For this review, use the dimensioned drawing (mm, ordinates from the lowest corner) and the shaded views. Give positions to 0.01 mm unless a question says otherwise; leave off trailing zeros. Order: outer loops, then holes, each group sorted by start corner. A loop starts at its lowest first (then second) coordinate and runs counter-clockwise, first axis right, second up.
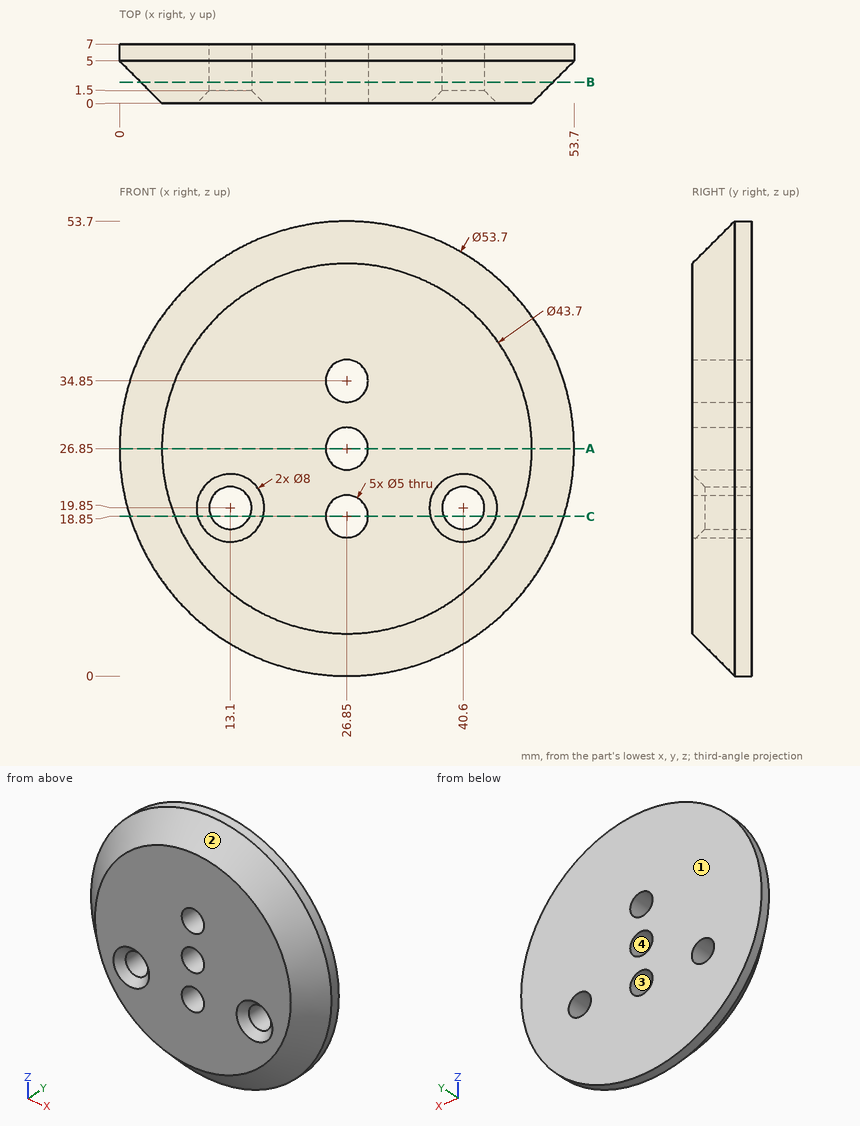
1. Take a section at A-A (z = 26.85). State the section outline as (x, y) points, then the cut area to 3 significant figures.
Recorded:
outline: (0, 5) - (5, 0) - (24.35, 0) - (24.35, 7) - (0, 7) - close; (29.35, 0) - (48.7, 0) - (53.7, 5) - (53.7, 7) - (29.35, 7) - close
area: 316 mm2
2. For pin 1 (3 mm diameter, centred on x = 26.85, z = 34.85, fed in from +Y), flat-tipped, find the tip position at first contact; note if it passes through.
Recorded:
pin 1: passes through
3. Take a section at B-B (y = 2.5). State the section outline as (x, z) points, then the cut area to 3 significant figures.
Recorded:
outline: circle Ø48.7 at (26.85, 26.85); hole circle Ø5 at (13.1, 19.85); hole circle Ø5 at (26.85, 18.85); hole circle Ø5 at (26.85, 26.85); hole circle Ø5 at (26.85, 34.85); hole circle Ø5 at (40.6, 19.85)
area: 1,760 mm2
4. For line 1 along Z through (x, y) = (26.85, 5.25); line 2 along X through (y, z) = (1, 17.5); line 3 along Y through (x, z) = (34, 47.5), list the stretches that pass through material, from the lowest coordinate up.
Recorded:
line 1: z = 0 to 16.35, 21.35 to 24.35, 29.35 to 32.35, 37.35 to 53.7
line 2: x = 6 to 11.24, 14.96 to 24.75, 28.95 to 38.74, 42.46 to 47.7
line 3: y = 0 to 7
5. Draft analysis for pull direction X (two halves, no side actions). For the marked faces 1, 2, 3 and 4, state which applies: pulls with the +X half, pulls with the -X half, needs draft (parallel to the pull), parting line crosses it, or undercut.
Recorded:
face 1: needs draft
face 2: parting line crosses it
face 3: undercut
face 4: undercut
6. Take a section at C-C (z = 18.85). State how many separate pieces and enclosed holes the cut face has, then the cut area to 3 significant figures.
Recorded:
separate pieces: 4
enclosed holes: 0
area: 229 mm2
